Geometry: final body of the model. Coordinates: model frame, mm. A direction names the side the tool comes from. Give positions to 0.01 mm unless a question says otherwise; leave off trailing zeros. Write each loop counter-clockwise with the first axis right and the second up, starting at its lowest first coordinate (ties: lowest second). Pieces come first, ordered by that corner, then holes.
```python
from build123d import *

# Parameters (mm, degrees)
SKETCH2_R           = 36.62
SKETCH2_R_2         = 29
BOSS_EXTRUDE1_DEPTH = 12.7
BOSS_EXTRUDE2_START = -12.7
SKETCH4_R           = 36.62
SKETCH4_R_2         = 27.305
BOSS_EXTRUDE2_DEPTH = 4.7625
SKETCH5_R           = 1.5875
CUT_EXTRUDE2_DEPTH  = 58.681962519
SKETCH6_R           = 63.5
CUT_EXTRUDE3_DEPTH  = 3.175


with BuildPart() as part:
    # Sketch2 → Boss-Extrude1 (new, symmetric)
    with BuildSketch(Plane(origin=(0, 0, 0), x_dir=(0, 0, -1), z_dir=(1, 0, 0))):
        Circle(SKETCH2_R)
        Circle(SKETCH2_R_2, mode=Mode.SUBTRACT)
    extrude(amount=BOSS_EXTRUDE1_DEPTH, both=True)

    # Sketch4 → Boss-Extrude2 (add, symmetric)
    with BuildSketch(Plane.ZY.offset(12.7).offset(BOSS_EXTRUDE2_START)):
        with Locations(Location((0, 0, 0), (0, 0, 180))):
            Circle(SKETCH4_R)
        with Locations(Location((0, 0, 0), (0, 0, 180))):
            Circle(SKETCH4_R_2, mode=Mode.SUBTRACT)
    extrude(amount=BOSS_EXTRUDE2_DEPTH, both=True)

    # Sketch5 → Cut-Extrude2 (cut, through all)
    with BuildSketch(Plane(origin=(12.7, 0, 0), x_dir=(0, 0, -1), z_dir=(1, 0, 0))):
        with Locations((31.75, 0)):
            Circle(SKETCH5_R)
        with Locations((27.49630657, -15.875)):
            Circle(SKETCH5_R)
        with Locations((15.875, -27.49630657)):
            Circle(SKETCH5_R)
        with Locations((0, -31.75)):
            Circle(SKETCH5_R)
        with Locations((-15.875, -27.49630657)):
            Circle(SKETCH5_R)
        with Locations((-27.49630657, -15.875)):
            Circle(SKETCH5_R)
        with Locations((-31.75, 0)):
            Circle(SKETCH5_R)
        with Locations((-27.49630657, 15.875)):
            Circle(SKETCH5_R)
        with Locations((-15.875, 27.49630657)):
            Circle(SKETCH5_R)
        with Locations((0, 31.75)):
            Circle(SKETCH5_R)
        with Locations((15.875, 27.49630657)):
            Circle(SKETCH5_R)
        with Locations((27.49630657, 15.875)):
            Circle(SKETCH5_R)
    extrude(amount=-CUT_EXTRUDE2_DEPTH, mode=Mode.SUBTRACT)

    # Sketch6 → Cut-Extrude3 (cut)
    with BuildSketch(Plane.ZY.offset(12.7)):
        Circle(SKETCH6_R)
    extrude(amount=-CUT_EXTRUDE3_DEPTH, mode=Mode.SUBTRACT)


solid = part.part
```
Item 1: Pin query (flat end, axial travel): pin 1 Ø12 at (x, y) = (-4.5, 27.5) entering from +Z; pin 2 Ø3 at (x, y) = (-4, -5) entering from -Z; pin 3 Ø1.5 at (x, z) = (-6.5, -19) entering from -Y. Return the tip coordinate at first contact, or that it passes through.
Found:
pin 1: stops at z = 29.64
pin 2: stops at z = -36.45
pin 3: stops at y = -31.75
Item 2: Section D-D, the plane z = 31.75. Return the cut outline in (x, y) (1 decimal).
Found:
outline: (-9.5, -18.2) - (12.7, -18.2) - (12.7, -1.6) - (-9.5, -1.6) - close; (-9.5, 1.6) - (12.7, 1.6) - (12.7, 18.2) - (-9.5, 18.2) - close
Item 3: Section A-A, the plane z = 0. Return the cut outline in (x, y) (1 decimal), plus the area to 3 significant figures.
Found:
outline: (-9.5, -36.6) - (12.7, -36.6) - (12.7, -33.3) - (-9.5, -33.3) - close; (-9.5, -30.2) - (12.7, -30.2) - (12.7, -29) - (4.8, -29) - (4.8, -27.3) - (-4.8, -27.3) - (-4.8, -29) - (-9.5, -29) - close; (-9.5, 29) - (-4.8, 29) - (-4.8, 27.3) - (4.8, 27.3) - (4.8, 29) - (12.7, 29) - (12.7, 30.2) - (-9.5, 30.2) - close; (-9.5, 33.3) - (12.7, 33.3) - (12.7, 36.6) - (-9.5, 36.6) - close
area: 230 mm2
Item 4: Pull-direction query (Y, two-part tool) for faces 4 (the face through (12.7, 27, 11)), 5 (the face through (1.432, -1.61, 36.585)), 6 (the face through (1.74, 33.09, -0.85)); classes: +Y half, -Y half, draft (parallel to the pull), parting line (faces both ways), or undercut.
Found:
face 4: draft
face 5: parting line
face 6: undercut
Item 5: Section C-C, the plane x = 10. State how many separate pieces and enclosed holes the cut face has, plus the area to 3 significant figures.
Found:
separate pieces: 1
enclosed holes: 13
area: 1,480 mm2
Item 6: Section B-B, the plane y = -3.5. Return the cut outline in (x, z) (1 decimal).
Found:
outline: (-9.5, -36.5) - (12.7, -36.5) - (12.7, -28.8) - (4.8, -28.8) - (4.8, -27.1) - (-4.8, -27.1) - (-4.8, -28.8) - (-9.5, -28.8) - close; (-9.5, 28.8) - (-4.8, 28.8) - (-4.8, 27.1) - (4.8, 27.1) - (4.8, 28.8) - (12.7, 28.8) - (12.7, 36.5) - (-9.5, 36.5) - close
Item 7: Reachability of faces 1 (the face through (1.74, -16.48, 26.03)), 2 (the face through (8.68, -25.73, -13.38)), 3 (the face through (-4.762, 26, -11)) from +Z, -Z, +X, -X, +Y, -Y: full face, straight path, thin tool, end or side. Return the list, or none.
Found:
face 1: +X, -X
face 2: +X
face 3: -X
Item 8: Line query: L1, parallel to Y at x = 3.75, z = 0 (1 decimal); L2, parallel to Y at x = 8, z = -15; L3, parallel to Z at x = 0.75, y = -16. Output: solid intervals per line, ascending.
Found:
L1: y = -36.6 to -33.3, -30.2 to -27.3, 27.3 to 30.2, 33.3 to 36.6
L2: y = -33.41 to -28.82, -26.17 to -24.82, 24.82 to 26.17, 28.82 to 33.41
L3: z = -32.94 to -29.08, -25.91 to -22.13, 22.13 to 25.91, 29.08 to 32.94
